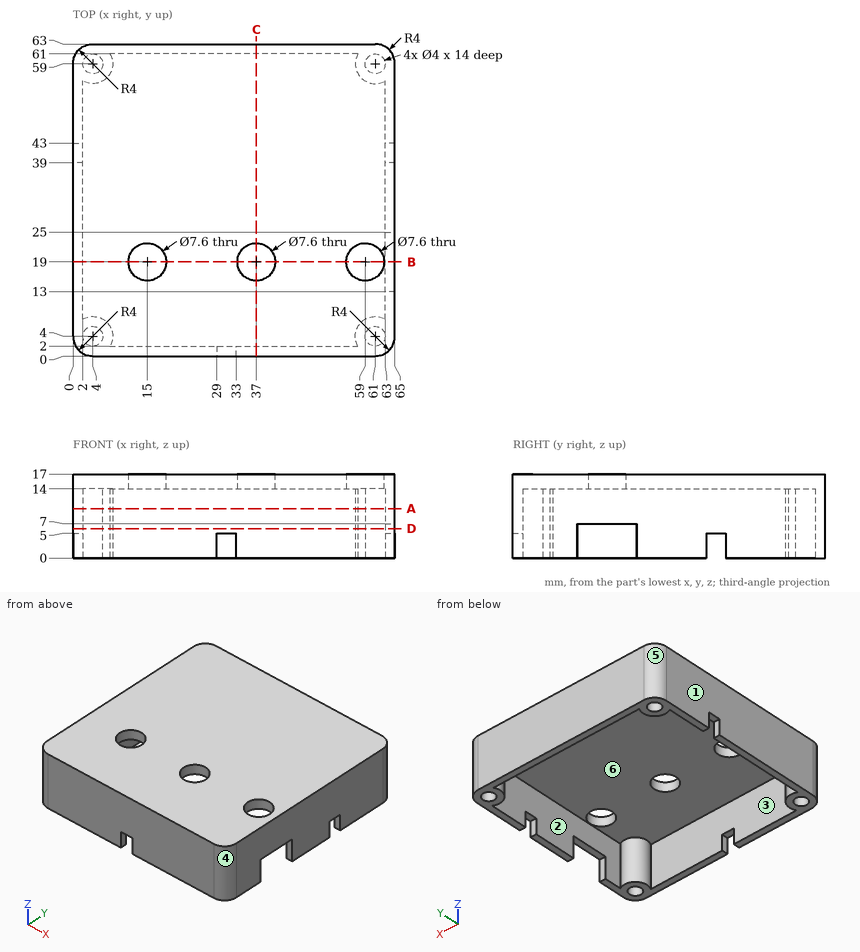
Source: three-view drawing plus pictorial views. Frame: mm from the lowest corner of the part. A direction names the side the tool comes from. Give positions to 0.01 mm unless a question says otherwise; leave off trailing zeros. Write each loop counter-clockwise with the first axis right and the second up, starting at its lowest first coordinate (ties: lowest second). Pieces come first, ordered by that corner, then holes.
(1) Cut plane C-C, the plane x = 37. Return loops of the section in (y, z).
(2) Cut plane B-B, the plane y = 19. Return loops of the section in (x, z), then the cut area to 3 significant figures.
(3) Mould query, pull axis X, two halves, no side actions, for the marked faces 1, 2, 3 and 4. Classes: released by +X, released by -X, zero draft, split by the parting line, or undercut.
(4) Access query for the marked faces 5 and 6. Directions: +Z, -Z, +X, -X, +Y, -Y. A direction counts if a zero-diameter tool reaches every point of the face in a straight line with its end or side. Return the directions, or none.
(5) Ray query, line 1 (Y direction, x = 4, z = 11.25); line 2 (X direction, y = 59, z = 10.5); line 3 (Y direction, x = 15, z = 14.9). Return the intervals inside material, ascending.
(6) First-contact query: P1, Ø2, axis at x = 60.5, y = 59, coming from the -Z side; P2, Ø0.6, axis at x = 30, y = 1, coming from the -Z side; P3, Ø0.6, axis at x = 64.5, z = 2, coming from the +Y side. Flat tips, straight axial feed; report the tip coordinate or a pass-through.
(7) Cut plane D-D, the plane z = 6. Return loops of the section in (x, y), then the cut area to 3 significant figures.
(8) Cut plane A-A, the plane z = 10. Return loops of the section in (x, y).
Values follow:
1. outline: (0, 0) - (2, 0) - (2, 14) - (15.2, 14) - (15.2, 17) - (0, 17) - close; (22.8, 14) - (61, 14) - (61, 0) - (63, 0) - (63, 17) - (22.8, 17) - close
2. outline: (0, 0) - (2, 0) - (2, 14) - (11.2, 14) - (11.2, 17) - (0, 17) - close; (18.8, 14) - (33.2, 14) - (33.2, 17) - (18.8, 17) - close; (40.8, 14) - (55.2, 14) - (55.2, 17) - (40.8, 17) - close; (62.8, 14) - (63, 14) - (63, 7) - (65, 7) - (65, 17) - (62.8, 17) - close
2. area: 169 mm2
3. face 1: released by -X
3. face 2: undercut
3. face 3: undercut
3. face 4: released by +X
4. face 5: +Z, -Z, -X, +Y
4. face 6: -Z
5. line 1: y = 0 to 2, 6 to 8, 55 to 57, 61 to 63
5. line 2: x = 0 to 2, 6 to 8, 57 to 59, 63 to 65
5. line 3: y = 0 to 15.2, 22.8 to 63
6. P1: stops at z = 14
6. P2: stops at z = 5
6. P3: stops at y = 61.4
7. outline: (0, 4) arc R4 ccw to (4, 0) - (61, 0) arc R4 ccw to (65, 4) - (65, 13) - (63, 13) - (63, 7.46) arc R4 ccw to (57.54, 2) - (7.46, 2) arc R4 ccw to (2, 7.46) - (2, 55.54) arc R4 ccw to (7.46, 61) - (57.54, 61) arc R4 ccw to (63, 55.54) - (63, 25) - (65, 25) - (65, 59) arc R4 ccw to (61, 63) - (4, 63) arc R4 ccw to (0, 59) - close; hole circle Ø4 at (4, 4); hole circle Ø4 at (4, 59); hole circle Ø4 at (61, 4); hole circle Ø4 at (61, 59)
7. area: 535 mm2
8. outline: (0, 4) arc R4 ccw to (4, 0) - (61, 0) arc R4 ccw to (65, 4) - (65, 59) arc R4 ccw to (61, 63) - (4, 63) arc R4 ccw to (0, 59) - close; hole circle Ø4 at (4, 4); hole (2, 7.46) arc R4 cw to (7.46, 2) - (57.54, 2) arc R4 cw to (63, 7.46) - (63, 55.54) arc R4 cw to (57.54, 61) - (7.46, 61) arc R4 cw to (2, 55.54) - close; hole circle Ø4 at (4, 59); hole circle Ø4 at (61, 4); hole circle Ø4 at (61, 59)
